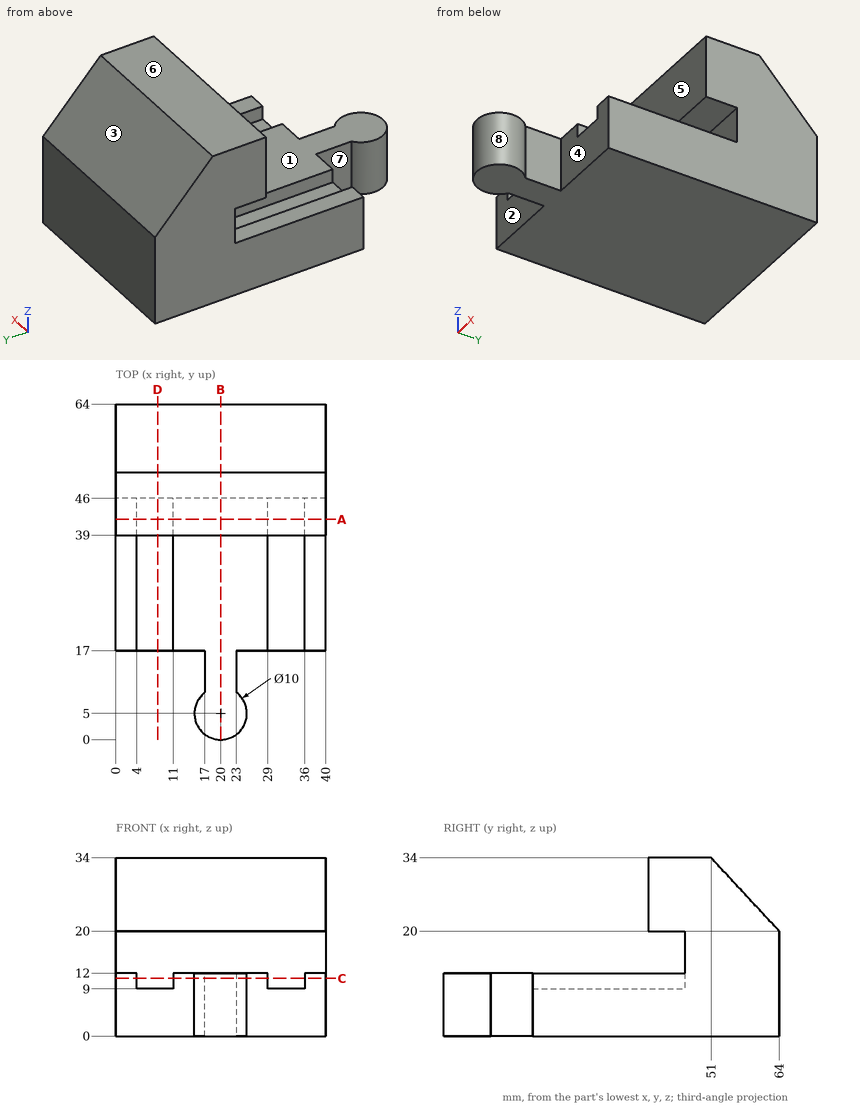
Verification items for this drawing (mm, ordinates from the low corner). A direction names the side the tool comes from. Give positions to 0.01 mm unless a question says otherwise; leave off trailing zeros. Write each loop counter-clockwise with the first axis right and the second up, starting at its lowest first coordinate (ties: lowest second). Pieces come first, ordered by that corner, then holes. Notation, with made-up numbers: (46, 68.5) - (100, 68.5) arc R24 cw to (100, 86.5) - close; hole circle Ø9 at (39.5, 68.5). An arc over 180 degrees is marked (long way). Answer as CSV lines item,"result". Start each with the question number.
1. Sectioned sample at A-A (y = 42). Record the boundary of the cut face in (x, z).
2. Set-up check for the marked faces 1, 2, 3 and 4: record each of +Z, -Z, +X, -X, +Y, -Y from which the full face is reachable in a straight line by a thin tool's end or side.
3. Sectioned sample at D-D (x = 8). Record the boundary of the cut face in (y, z), then the cut area to 3 significant figures.
4. Draft check along Y on the marked faces 5, 6, 7 and 8. Enter one of: pulls with the +Y half, pulls with the -Y half, needs draft (parallel to the pull), parting line crosses it, or undercut.
5. Thickness scan on line 1 (Z direction, x = 5, y = 41.5); line 2 (Y direction, x = 30.5, z = 4); line 3 (Z direction, x = 32, y = 34). Record the ranges inside material, lowest first.
6. Sectioned sample at B-B (x = 20). Record the boundary of the cut face in (y, z), then the cut area to 3 significant figures.
7. Depth check by flat-ended pin: pin 1 (10 mm diameter, centred on x = 27, z = 30.5, fed in from +Y); pin 2 (2 mm diameter, centred on x = 7, y = 37, fed in from +Z); pin 3 (2 mm diameter, centred on x = 1.5, y = 35, fed in from +Z). Enter the tip coordinate at first touch or a pass-through.
8. Sectioned sample at C-C (z = 11). Record the boundary of the cut face in (x, y), then the cut area to 3 significant figures.
Derived:
1,outline,"(0, 0) - (40, 0) - (40, 12) - (36, 12) - (36, 9) - (29, 9) - (29, 12) - (11, 12) - (11, 9) - (4, 9) - (4, 12) - (0, 12) - close; (0, 20) - (40, 20) - (40, 34) - (0, 34) - close"
2,face 1,"+X, -X, -Y"
2,face 2,"+Z, -Z, -X"
2,face 3,"+Z, +X, -X, +Y"
2,face 4,"+Z, -Z, +X"
3,outline,"(17, 0) - (64, 0) - (64, 20) - (51, 34) - (39, 34) - (39, 20) - (46, 20) - (46, 9) - (17, 9) - close"
3,area,"880 mm²"
4,face 5,"pulls with the -Y half"
4,face 6,"needs draft"
4,face 7,"undercut"
4,face 8,"undercut"
5,line 1,"0 to 9, 20 to 34"
5,line 2,"17 to 64"
5,line 3,"0 to 9"
6,outline,"(0, 0) - (64, 0) - (64, 20) - (51, 34) - (39, 34) - (39, 20) - (46, 20) - (46, 12) - (0, 12) - close"
6,area,"1,170 mm²"
7,pin 1,"y = 58.89"
7,pin 2,"z = 9"
7,pin 3,"z = 12"
8,outline,"(0, 17) - (4, 17) - (4, 46) - (11, 46) - (11, 17) - (17, 17) - (17, 9) arc R5 ccw (long way) to (23, 9) - (23, 17) - (29, 17) - (29, 46) - (36, 46) - (36, 17) - (40, 17) - (40, 64) - (0, 64) - close"
8,area,"1,600 mm²"
